```python
from build123d import *

# Parameters (mm, degrees)
F1_DEPTH = 76.2
F2_T     = -2.54


with BuildPart() as f1:
    # F0 (on Top) → F1 (new body)
    with BuildSketch(Plane.XY):
        with BuildLine():
            Line((203.2, 0), (63.5, 0))
            Line((63.5, 0), (63.5, -63.5))
            Line((63.5, -63.5), (0, -63.5))
            Line((0, -63.5), (0, -609.6))
            Line((0, -609.6), (38.1, -609.6))
            ThreePointArc((38.1, -609.6), (80.202006, -312.165024), (203.2, -38.1))
            Line((203.2, -38.1), (203.2, 0))
        make_face()
    extrude(amount=-F1_DEPTH)

    # F2
    f2_openings = [f1.faces().sort_by_distance(p)[0] for p in [
        (66.483993, -223.719229, -76.2),
        (80.202006, -312.165024, -38.1),
        (31.75, -63.5, -38.1),
        (63.5, -31.75, -38.1),
    ]]
    offset(amount=F2_T, openings=f2_openings)


solid = f1.part
```
Check sheet for the modelled part. Datum: model origin and axes. Units: mm. A direction names the side the tool comes from. Round coordinates to 2 decimals unless told otherwise and drop trailing zeros. Order: outer loops, then holes, each group sorted by start corner. A loop starts at its lowest first (then second) coordinate and runs counter-clockwise, first axis right, second up.
1) Section check B-B (x = 127.5). Record the boundary of the cut face in (y, z).
2) Scan lines: line 1 (Z direction, x = 61.5, y = -194.5); line 2 (X direction, y = -234, z = -7). Record each from-to range of solid material in increasing order.
3) Section check C-C (y = -244.5). Record the boundary of the cut face in (x, z), and give its area (3 significant figures).
4) Section check D-D (x = 47.5). Record the boundary of the cut face in (y, z), and give its area (3 significant figures).
5) Section check A-A (z = -47). Record the boundary of the cut face in (x, y).
6) Tool access check on faces 1 (the flat face through (78, -233, -2.54)), 2 (the flat face through (1, -63.5, -21)), 3 (the cylindrical face through (79.81, -313.52, -1.23)), 4 (the flat face through (133, -2.54, -39)), 5 (the flat face through (20, -607.06, -39)). Record the directions out of +Z, -Z, +X, -X, +Y, -Y that give a thin tool (end or side, any length) a straight path to the whole face; none if there is none.
7) Go/stop test with flat-tipped pins: pin 1 Ø5 at (x, y) = (121.5, -154.5) entering from -Z; pin 2 Ø4 at (y, z) = (-103, -52.5) entering from +X. Record where each tip stops, or that it passes through.
Result:
1. outline: (-181.09, -2.54) - (-2.54, -2.54) - (-2.54, -76.2) - (0, -76.2) - (0, 0) - (-181.09, 0) - close
2. line 1: z = -2.54 to 0
2. line 2: x = 0 to 2.54
3. outline: (0, -76.2) - (2.54, -76.2) - (2.54, -2.54) - (102.21, -2.54) - (102.21, 0) - (0, 0) - close
3. area: 447 mm2
4. outline: (-467.97, -2.54) - (-63.5, -2.54) - (-63.5, 0) - (-467.97, 0) - close
4. area: 1,030 mm2
5. outline: (0, -609.6) - (38.1, -609.6) arc R1071.68 cw to (38.1, -607.06) - (2.54, -607.06) - (2.54, -63.5) - (0, -63.5) - close; (63.5, -2.54) - (200.66, -2.54) - (200.66, -42.15) arc R1071.68 cw to (203.2, -38.1) - (203.2, 0) - (63.5, 0) - close
6. face 1: -Z
6. face 2: +Z, -Z, -X, +Y
6. face 3: +Z, -Z, +X, -Y
6. face 4: -Z, -X, -Y
6. face 5: -Z, +X, +Y
7. pin 1: stops at z = -2.54
7. pin 2: stops at x = 2.54
